Autodesk Fusion 360 part; units mm, degrees
sketch "Sketch1" plane through (0, 0, 0) normal (0, 1, 0) x (1, 0, 0)
  line L0 (0, -12.5) -> (23, -12.5)
  line L1 (25, -10.5) -> (25, 10.5)
  line L2 (23, 12.5) -> (0, 12.5)
  line L3 (0, -12.5) -> (-23, -12.5)
  line L4 (-25, -10.5) -> (-25, 10.5)
  line L5 (-23, 12.5) -> (0, 12.5)
  arc A0 (-25, -10.5) -> (-23, -12.5) centre (-23, -10.5) ccw
  arc A1 (23, -12.5) -> (25, -10.5) centre (23, -10.5) ccw
  arc A2 (-23, 12.5) -> (-25, 10.5) centre (-23, 10.5) ccw
  line L6 (-23, 10.5) -> (0, 10.5)
  line L7 (23, 10.5) -> (0, 10.5)
  line L8 (23, -10.5) -> (23, 10.5)
  line L9 (0, -10.5) -> (23, -10.5)
  line L10 (0, -10.5) -> (-23, -10.5)
  line L11 (-23, -10.5) -> (-23, 10.5)
  arc A3 (25, 10.5) -> (23, 12.5) centre (23, 10.5) ccw
  point P0 (25, -12.5)
  dimension "d1" = 12.5
  dimension "d2" = 25
  dimension "d3" = 25
  dimension "d4" = 2
  dimension "d5" = 2
  dimension "d6" = 2
  dimension "d7" = 2
extrude "Extrude1" add sketch "Sketch1" along normal blind 700
Input: part model. Units: mm. Frame: model coordinates. A direction names the side the tool comes from. Give positions to 0.01 mm unless a question says otherwise; leave off trailing zeros. Write each loop counter-clockwise with the first axis right and the second up, starting at its lowest first coordinate (ties: lowest second). Pieces come first, ordered by that corner, then holes. Notation, with made-up numbers: M 89.25,79 L 132.25,79 A17 ccw 132.25,83 Z; hole C 41,25.25 d10. An arc over 180 degrees is marked long. Use one line per item in the form item = value.
1. Ray query, L1, parallel to Z at x = -18.5, y = 659.5; L2, parallel to X at y = 200.5, z = 5. Return the intervals inside material, ascending.
Outcome:
L1 = -12.5 to -10.5, 10.5 to 12.5
L2 = -25 to -23, 23 to 25
2. Cut plane C-C on y = 380. Return loops of the section in (x, z).
Outcome:
outline = M -25,-10.5 A2 ccw -23,-12.5 L 23,-12.5 A2 ccw 25,-10.5 L 25,10.5 A2 ccw 23,12.5 L -23,12.5 A2 ccw -25,10.5 Z; hole M -23,-10.5 L 23,-10.5 L 23,10.5 L -23,10.5 Z
3. Cut plane B-B on z = 0. Return loops of the section in (x, y).
Outcome:
outline = M -25,0 L -23,0 L -23,700 L -25,700 Z; M 23,0 L 25,0 L 25,700 L 23,700 Z
4. Reachability of faces 1 (the face through (23, 345, 0)), 2 (the face through (0, 345, -12.5)) from +Z, -Z, +X, -X, +Y, -Y: full face, straight path, thin tool, end or side. Return the list, or none.
Outcome:
face_1 = +Y, -Y
face_2 = -Z, +X, -X, +Y, -Y
5. Cut plane A-A on x = -0.5. Return loops of the section in (y, z).
Outcome:
outline = M 0,-12.5 L 700,-12.5 L 700,-10.5 L 0,-10.5 Z; M 0,10.5 L 700,10.5 L 700,12.5 L 0,12.5 Z
6. First-contact query: P1, Ø5, axis at x = -16, z = -6, coming from the +Y side. Flat tip, straight axial feed; report the tip coordinate or a pass-through.
Outcome:
P1 = through
